```python
from build123d import *

# Parameters (mm, degrees)
FUROS_GUIA_COM_10_0MM1_D           = 10
FUROS_GUIA_COM_10_0MM1_CSINK_D     = 10.05
FUROS_GUIA_COM_10_0MM1_CSINK_ANGLE = 90
FILETE1_R                          = 2
CHANFRO4_SIZE                      = 1
CHANFRO6_SIZE                      = 1


with BuildPart() as part:
    # Esboço1 → Revolução1 (revolve)
    with BuildSketch(Plane.XY):
        Polygon((0, 0), (0, 25), (15, 25), (15, 15), (60, 15), (60, 10), (110, 10), (110, 0), align=None)
    revolve(axis=Axis((110, 0, 0), (-1, 0, 0)))

    # Furos-guia com Ø10.0mm1 (through all)
    with Locations(Plane(origin=(110, 0, 0), x_dir=(0, 0, -1), z_dir=(1, 0, 0))):
        with Locations((0, 0)):
            CounterSinkHole(FUROS_GUIA_COM_10_0MM1_D / 2, FUROS_GUIA_COM_10_0MM1_CSINK_D / 2, counter_sink_angle=FUROS_GUIA_COM_10_0MM1_CSINK_ANGLE)

    # Filete1
    filete1_edges = [part.edges().sort_by_distance(p)[0] for p in [
        (60, -10, 0),
        (15, -15, 0),
    ]]
    fillet(filete1_edges, radius=FILETE1_R)

    # Chanfro4
    chanfro4_edges = [part.edges().sort_by_distance(p)[0] for p in [
        (110, -10, 0),
        (60, -15, 0),
        (0, -25, 0),
    ]]
    chamfer(chanfro4_edges, length=CHANFRO4_SIZE)

    # Chanfro6
    chanfro6_edges = [part.edges().sort_by_distance(p)[0] for p in [
        (0, 0, -5),
    ]]
    chamfer(chanfro6_edges, length=CHANFRO6_SIZE)


solid = part.part
```
The listing builds one solid part. Answer for the finished solid, in the listing's coordinates (mm). A direction names the side the tool comes from. Give positions to 0.01 mm unless a question says otherwise; leave off trailing zeros. Order: outer loops, then holes, each group sorted by start corner. A loop starts at its lowest first (then second) coordinate and runs counter-clockwise, first axis right, second up. Notation, with made-up numbers: M 59.5,65.5 L 93.5,65.5 A31 ccw 93.5,101.5 Z; hole C -6.75,53 d10. An arc over 180 degrees is marked long. Put each result on its own line as item: value. Start each with the question number.
Item 1: For a pull along Y with two mould halves and no side action, classify faces 3 (the face through (85.83, -2.17, 9.76)), 4 (the face through (54.72, -4.88, -1.08)), 5 (the face through (15, -5.9, 16.3)) as +Y half, -Y half, draft (parallel to the pull), parting line (faces both ways), or undercut.
Item 2: Which of the six approach directions +Z, -Z, +X, -X, +Y, -Y give full straight-line access (tool end or side, diameter ignored) to faces 1 (the face through (38.294, -14.985, -0.66)), 2 (the face through (0, -5, 5))?
Item 3: The part is cut by section C-C, the plane x = 24.5. Determine the outline of the cut face in (y, z).
Item 4: Find the intervals of material crossed by line 1 along Y through (x, z) = (39, 0); line 2 along Z through (x, y) = (82, 0), in increasing order.
Item 5: The part is cut by section D-D, the plane x = 72.5. Determine the outline of the cut face in (y, z), and give its area (3 significant figures).
Item 6: Flat-ended cylindrical pins translate along their axes: P1, Ø3, axis at x = 17, z = -4.5, coming from the +Y side; P2, Ø12, axis at y = 13, z = -15, coming from the +X side; P3, Ø5, axis at y = 13, z = 3, coming from the +X side. Find the tip coordinate at first contact, or state that the pin passes through.
Answer key:
1. face 3: parting line
1. face 4: undercut
1. face 5: draft
2. face 1: +X
2. face 2: +Z, -Z, -X, +Y, -Y
3. outline: C 0,0 d30; hole C 0,0 d10
4. line 1: y = -15 to -5, 5 to 15
4. line 2: z = -10 to -5, 5 to 10
5. outline: C 0,0 d20; hole C 0,0 d10
5. area: 236 mm²
6. P1: stops at y = 15.07
6. P2: stops at x = 60
6. P3: stops at x = 60.37
